```python
from build123d import *

# Parameters (mm, degrees)
SKETCH1_R                                       = 50
SKETCH1_R_2                                     = 11.1125
BOSS_EXTRUDE1_DEPTH                             = 5
CSK_FOR_M3_FLAT_HEAD_MACHINE_SCREW1_D           = 3.4
CSK_FOR_M3_FLAT_HEAD_MACHINE_SCREW1_CSINK_D     = 6.3
CSK_FOR_M3_FLAT_HEAD_MACHINE_SCREW1_CSINK_ANGLE = 90
CIRPATTERN1_COUNT                               = 4
CHAMFER1_SIZE                                   = 2


with BuildPart() as part:
    # Sketch1 → Boss-Extrude1 (new body)
    with BuildSketch(Plane(origin=(0, 0, 0), x_dir=(1, 0, 0), z_dir=(0, 1, 0))):
        with Locations(Location((0, 0, 0), (0, 0, 270))):
            Circle(SKETCH1_R)
        with Locations(Location((0, 0, 0), (0, 0, 270))):
            Circle(SKETCH1_R_2, mode=Mode.SUBTRACT)
    extrude(amount=BOSS_EXTRUDE1_DEPTH)

    # CSK for M3 Flat Head Machine Screw1 (through all)
    with Locations(Plane(origin=(0, 5, 0), x_dir=(1, 0, 0), z_dir=(0, 1, 0))):
        with Locations((0, 42.5)):
            csk_for_m3_flat_head_machine_screw1 = CounterSinkHole(CSK_FOR_M3_FLAT_HEAD_MACHINE_SCREW1_D / 2, CSK_FOR_M3_FLAT_HEAD_MACHINE_SCREW1_CSINK_D / 2, counter_sink_angle=CSK_FOR_M3_FLAT_HEAD_MACHINE_SCREW1_CSINK_ANGLE)

    # CirPattern1: CSK for M3 Flat Head Machine Screw1 ×4 about axis
    cirpattern1_axis = Axis((0, 0, 0), (0, 1, 0))
    for i in range(1, CIRPATTERN1_COUNT):
        add(csk_for_m3_flat_head_machine_screw1.rotate(cirpattern1_axis, i * 360 / CIRPATTERN1_COUNT), mode=Mode.SUBTRACT)

    # Chamfer1
    chamfer1_edges = [part.edges().sort_by_distance(p)[0] for p in [
        (0, 5, -50),
    ]]
    chamfer(chamfer1_edges, length=CHAMFER1_SIZE)


solid = part.part
```
Geometry: final body of the model. Coordinates: model frame, mm. Coordinates: 2 decimals unless noted, no trailing zeros. Order: outer loops, then holes, each group sorted by start corner. A loop starts at its lowest first (then second) coordinate and runs counter-clockwise, first axis right, second up. Notation, with made-up numbers: (51, -18) -> (71, -18) arc R11 ccw to (71, -12) -> close; hole circle Ø6 at (20.25, -32.75). An arc over 180 degrees is marked (long way). Use CSV: the item, a comma, the result in double quotes.
1) Line query: line 1 (X direction, y = 1.6, z = 0); line 2 (X direction, y = 3.55, z = 0); line 3 (Z direction, x = 14, y = 0.3). Output: solid intervals per line, ascending.
Findings:
line 1,"x = -50 to -44.2, -40.8 to -11.11, 11.11 to 40.8, 44.2 to 50"
line 2,"x = -49.45 to -44.2, -40.8 to -11.11, 11.11 to 40.8, 44.2 to 49.45"
line 3,"z = -48 to 48"
2) Section B-B on y = 1.35. Output: boundary loops of the cut face in (x, z) (1 decimal), then the cut area to 3 significant figures.
Findings:
outline,"circle Ø100 at (0, 0); hole circle Ø3.4 at (-42.5, 0); hole circle Ø22.2 at (0, 0); hole circle Ø3.4 at (0, -42.5); hole circle Ø3.4 at (0, 42.5); hole circle Ø3.4 at (42.5, 0)"
area,"7,430 mm^2"
3) Pin query (flat end, axial travel): pin 1 Ø1 at (x, z) = (-17.5, 36.5) entering from -Y; pin 2 Ø4 at (x, z) = (0, -42.5) entering from +Y; pin 3 Ø1.5 at (y, z) = (4, -8.5) entering from +X; pin 4 Ø2.5 at (x, z) = (0, 42.5) entering from -Y. Return the tip coordinate at first contact, or that it passes through.
Findings:
pin 1,"stops at y = 0"
pin 2,"stops at y = 3.85"
pin 3,"stops at x = 49.03"
pin 4,"passes through"
4) Section A-A on x = 0. Output: boundary loops of the cut face in (y, z), then the cut area to 3 significant figures.
Findings:
outline,"(0, -50) -> (3, -50) -> (5, -48) -> (5, -45.65) -> (3.55, -44.2) -> (0, -44.2) -> close; (0, -40.8) -> (3.55, -40.8) -> (5, -39.35) -> (5, -11.11) -> (0, -11.11) -> close; (0, 11.11) -> (5, 11.11) -> (5, 39.35) -> (3.55, 40.8) -> (0, 40.8) -> close; (0, 44.2) -> (3.55, 44.2) -> (5, 45.65) -> (5, 48) -> (3, 50) -> (0, 50) -> close"
area,"347 mm^2"
5) Mould query, pull axis X, two halves, no side actions, for faces 1 (the flat face through (11.3, 5, -0.7)), 2 (the cylindrical face through (15.02, 1.48, 47.69)), 3 (the cylindrical face through (-0.37, 1.75, 40.84)). Classes: +X half, -X half, draft (parallel to the pull), parting line (faces both ways), or undercut.
Findings:
face 1,"draft"
face 2,"parting line"
face 3,"undercut"
